```python
from build123d import *

# Parameters (mm, degrees)
BOSS_EXTRUDE1_DEPTH            = 3.175
F_3_16_0_1875_DIAMETER_HOLE1_D = 4.7625
FILLET1_R                      = 0.635


with BuildPart() as part:
    # Sketch1 → Boss-Extrude1 (new body)
    with BuildSketch(Plane.XY):
        Polygon((19.05, 12.7), (-19.05, 12.7), (-22.225, 9.525), (-22.225, -9.525), (-19.05, -12.7), (19.05, -12.7), (22.225, -9.525), (22.225, 9.525), align=None)
    extrude(amount=BOSS_EXTRUDE1_DEPTH)

    # 3/16 (0.1875) Diameter Hole1 (through all)
    with Locations(Plane.XY.offset(3.175)):
        with Locations((15.875, 0), (-15.875, 0)):
            Hole(F_3_16_0_1875_DIAMETER_HOLE1_D / 2)

    # Fillet1
    fillet1_edges = [part.edges().sort_by_distance(p)[0] for p in [
        (-20.6375, 11.1125, 3.175),
        (0, 12.7, 0),
        (20.6375, 11.1125, 0),
        (-22.225, 0, 3.175),
        (-20.6375, -11.1125, 3.175),
        (0, -12.7, 3.175),
        (20.6375, -11.1125, 3.175),
        (22.225, 0, 3.175),
        (-13.49375, 0, 3.175),
        (-13.49375, 0, 0),
        (18.25625, 0, 3.175),
        (18.25625, 0, 0),
        (20.6375, 11.1125, 3.175),
        (0, 12.7, 3.175),
        (22.225, 0, 0),
        (20.6375, -11.1125, 0),
        (0, -12.7, 0),
        (-20.6375, -11.1125, 0),
        (-22.225, 0, 0),
        (-20.6375, 11.1125, 0),
    ]]
    fillet(fillet1_edges, radius=FILLET1_R)


solid = part.part
```
Geometry check sheet. Reference: the model listing, model coordinates, mm. Give positions to 0.01 mm unless a question says otherwise; leave off trailing zeros. Order: outer loops, then holes, each group sorted by start corner. A loop starts at its lowest first (then second) coordinate and runs counter-clockwise, first axis right, second up. Notation, with made-up numbers: (43.5, -12) - (78.5, -12) arc R20 cw to (78.5, 15) - close; hole circle Ø5 at (-35.5, 1). An arc over 180 degrees is marked (long way). Answer in a Markdown table with one row per item. Add a question column.
Q1. Material ranges on probe 1 along X at (y, z) = (2, 1.25) (3 decimals); probe 2 along X at (y, z) = (-5, 3); probe 3 along Y at (x, z) = (18, 0.45), recorded low to high. Write a range as from..to.
Q2. Cross-section at A-A, the plane y = 0. Enter the section's corners in (x, z) (3 decimals).
Q3. Mould release check, pull along Y, two halves, no side actions. Record for faces 1 (the cylindrical face through (20.52, -10.96, 0.18)), 2 (the cylindrical face through (13.6, 0.7, 1.6)), 3 (the flat face through (20.66, 11.09, 1.57)): pulls with the +Y half, pulls with the -Y half, needs draft (parallel to the pull), parting line crosses it, or undercut.
Check values:
| question | item | result |
|---|---|---|
| 1 | probe 1 | x = -22.225..-17.167, -14.583..14.583, 17.167..22.225 |
| 1 | probe 2 | x = -22.03..22.03 |
| 1 | probe 3 | y = -12.67..-1.13, 1.13..12.67 |
| 2 | outline | (-22.225, 0.635) arc R0.635 ccw to (-21.59, 0) - (-18.891, 0) arc R0.635 ccw to (-18.256, 0.635) - (-18.256, 2.54) arc R0.635 ccw to (-18.891, 3.175) - (-21.59, 3.175) arc R0.635 ccw to (-22.225, 2.54) - close; (-13.494, 0.635) arc R0.635 ccw to (-12.859, 0) - (12.859, 0) arc R0.635 ccw to (13.494, 0.635) - (13.494, 2.54) arc R0.635 ccw to (12.859, 3.175) - (-12.859, 3.175) arc R0.635 ccw to (-13.494, 2.54) - close; (18.256, 0.635) arc R0.635 ccw to (18.891, 0) - (21.59, 0) arc R0.635 ccw to (22.225, 0.635) - (22.225, 2.54) arc R0.635 ccw to (21.59, 3.175) - (18.891, 3.175) arc R0.635 ccw to (18.256, 2.54) - close |
| 3 | face 1 | pulls with the -Y half |
| 3 | face 2 | undercut |
| 3 | face 3 | pulls with the +Y half |
